```python
from build123d import *

# Parameters (mm, degrees)
SKETCH1_W           = 150
SKETCH1_H           = 110
BOSS_EXTRUDE1_DEPTH = 4
SKETCH2_W           = 96
SKETCH2_H           = 100
BOSS_EXTRUDE2_DEPTH = 100
FILLET1_R           = 3
SKETCH4_R           = 5
CUT_EXTRUDE1_DEPTH  = 15
SKETCH5_W           = 147
SKETCH5_H           = 147
BOSS_EXTRUDE3_DEPTH = 4
SKETCH6_R           = 2.5
CUT_EXTRUDE2_DEPTH  = 5
FILLET2_R           = 8


with BuildPart() as part:
    # Sketch1 → Boss-Extrude1 (new body)
    with BuildSketch(Plane(origin=(0, 0, 0), x_dir=(1, 0, 0), z_dir=(0, 1, 0))):
        with Locations((75, 55)):
            Rectangle(SKETCH1_W, SKETCH1_H)
    extrude(amount=BOSS_EXTRUDE1_DEPTH)

    # Sketch2 → Boss-Extrude2 (add)
    with BuildSketch(Plane(origin=(0, 4, 0), x_dir=(1, 0, 0), z_dir=(0, 1, 0))):
        with Locations((75, 55)):
            Rectangle(SKETCH2_W, SKETCH2_H)
    extrude(amount=BOSS_EXTRUDE2_DEPTH)

    # Fillet1
    fillet1_edges = [part.edges().sort_by_distance(p)[0] for p in [
        (150, 4, -55),
        (27, 54, -105),
        (27, 54, -5),
        (75, 4, -110),
        (123, 54, -5),
        (123, 54, -105),
        (27, 104, -55),
        (75, 104, -5),
        (123, 104, -55),
        (75, 104, -105),
        (0, 4, -55),
        (75, 4, 0),
    ]]
    fillet(fillet1_edges, radius=FILLET1_R)

    # Sketch4 → Cut-Extrude1 (cut)
    with BuildSketch(Plane(origin=(0, 104, 0), x_dir=(1, 0, 0), z_dir=(0, 1, 0))):
        with Locations((75, 55)):
            Circle(SKETCH4_R)
    extrude(amount=-CUT_EXTRUDE1_DEPTH, mode=Mode.SUBTRACT)

    # Sketch5 → Boss-Extrude3 (add)
    with BuildSketch(Plane.XZ):
        with Locations((75, -55)):
            Rectangle(SKETCH5_W, SKETCH5_H)
    extrude(amount=BOSS_EXTRUDE3_DEPTH)

    # Sketch6 → Cut-Extrude2 (cut, through all)
    with BuildSketch(Plane(origin=(0, 0, 0), x_dir=(1, 0, 0), z_dir=(0, 1, 0))):
        with Locations((11.5, 118.5)):
            Circle(SKETCH6_R)
        with Locations((138.5, 118.5)):
            Circle(SKETCH6_R)
        with Locations((11.5, -8.5)):
            Circle(SKETCH6_R)
        with Locations((138.5, -8.5)):
            Circle(SKETCH6_R)
    extrude(amount=-CUT_EXTRUDE2_DEPTH, mode=Mode.SUBTRACT)

    # Fillet2
    fillet2_edges = [part.edges().sort_by_distance(p)[0] for p in [
        (1.5, -2, 18.5),
        (1.5, -2, -128.5),
        (148.5, -2, -128.5),
        (148.5, -2, 18.5),
    ]]
    fillet(fillet2_edges, radius=FILLET2_R)


solid = part.part
```
Part model, mm, in its own coordinate system. A direction names the side the tool comes from. Round coordinates to 2 decimals unless told otherwise and drop trailing zeros. Loops run counter-clockwise (first coordinate to the right, second up) from the corner with the lowest first, then second, coordinate; pieces in that order, holes last. Notation, with made-up numbers: (10, 51) -> (21, 51) arc R18 ccw to (21, 83) -> close; hole circle Ø2 at (0.5, 69). An arc over 180 degrees is marked (long way). Use CSV: the item, a comma, the result in double quotes. Start each with the question number.
1) Which spindle directions (+Z, -Z, +X, -X, +Y, -Y) get a long thin tool onto all of the face, cutting with end or side? Do faces 1 (the flat face through (74, 0, 9)), 2 (the flat face through (1.5, -2, -56)), 3 (the flat face through (74, 0, -119)), 4 (the cylindrical face through (78, 97, -59)), 5 (the flat face through (148.5, -2, -56)). Say none if no direction does.
2) Cut at A-A, the plane x = 11.5. Write the cut outline in (y, z).
3) Drop flat-ended pins along their axis: P1, Ø1.5, axis at x = 132.5, z = -51, coming from the +Y side; P2, Ø6, axis at x = 138.5, z = -118.5, coming from the -Y side; P3, Ø20.5, axis at x = 103.5, z = -122, coming from the +Y side; P4, Ø2, axis at x = 59, y = 63, coming from the +Z side. Give the stop position or say it passes through.
4) Wall check: L1, parallel to X at y = -2.05, z = -118.5; L2, parallel to Z at x = 138.5, y = -1.2; L3, parallel to X at y = 96, z = -55. Give the ranges that are in metal, low to high. Write a range as [from, to].
5) Cut at C-C, the plane x = 75. Write the cut outline in (y, z).
6) Pull direction Z, two halves, no side cores. Call faces 6 (the flat face through (27, 52, -54)), 7 (the cylindrical face through (140.885, -1.972, -119.251)), 8 (the flat face through (74, 52, -105)): +Z half, -Z half, draft (parallel to the pull), parting line (faces both ways), or undercut.
7) Cut at D-D, the plane z = -47. Write the cut outline in (x, y), plus the area to 3 significant figures.
8) Cut at B-B, the plane z = 8.5. Write the cut outline in (x, y), plus the area to 3 significant figures.
Determined:
1,face 1,"+Z, +X, -X, +Y"
1,face 2,"+Z, -Z, -X, -Y"
1,face 3,"-Z, +X, -X, +Y"
1,face 4,"+Y"
1,face 5,"+Z, -Z, +X, -Y"
2,outline,"(-4, -128.5) -> (0, -128.5) -> (0, -121) -> (-4, -121) -> close; (-4, -116) -> (0, -116) -> (0, -110) -> (1, -110) arc R3 ccw to (4, -107) -> (4, -3) arc R3 ccw to (1, 0) -> (0, 0) -> (0, 6) -> (-4, 6) -> close; (-4, 11) -> (0, 11) -> (0, 18.5) -> (-4, 18.5) -> close"
3,P1,"stops at y = 4"
3,P2,"stops at y = -4"
3,P3,"stops at y = 0"
3,P4,"stops at z = -5"
4,L1,"x = [1.5, 9], [14, 136], [141, 148.5]"
4,L2,"z = [-128.5, -121], [-116, 6], [11, 18.5]"
4,L3,"x = [27, 70], [80, 123]"
5,outline,"(-4, -128.5) -> (0, -128.5) -> (0, -110) -> (1, -110) arc R3 ccw to (4, -107) -> (4, -105) -> (101, -105) arc R3 ccw to (104, -102) -> (104, -60) -> (89, -60) -> (89, -50) -> (104, -50) -> (104, -8) arc R3 ccw to (101, -5) -> (4, -5) -> (4, -3) arc R3 ccw to (1, 0) -> (0, 0) -> (0, 18.5) -> (-4, 18.5) -> close"
6,face 6,"draft"
6,face 7,"undercut"
6,face 8,"-Z half"
7,outline,"(0, 0) -> (1.5, 0) -> (1.5, -4) -> (148.5, -4) -> (148.5, 0) -> (150, 0) -> (150, 1) arc R3 ccw to (147, 4) -> (123, 4) -> (123, 101) arc R3 ccw to (120, 104) -> (30, 104) arc R3 ccw to (27, 101) -> (27, 4) -> (3, 4) arc R3 ccw to (0, 1) -> close"
7,area,"10,800 mm2"
8,outline,"(1.5, -4) -> (9, -4) -> (9, 0) -> (1.5, 0) -> close; (14, -4) -> (136, -4) -> (136, 0) -> (14, 0) -> close; (141, -4) -> (148.5, -4) -> (148.5, 0) -> (141, 0) -> close"
8,area,"548 mm2"
